```python
from build123d import *

# Parameters (mm, degrees)
SKETCH1_R             = 60.5
BOSS_EXTRUDE1_DEPTH   = 4
SKETCH2_R             = 12
CUT_EXTRUDE1_DEPTH    = 4
F_3_0MM_DOWEL_HOLE1_D = 3
SKETCH6_W             = 4
SKETCH6_H             = 46
CUT_EXTRUDE2_DEPTH    = 4


with BuildPart() as part:
    # Sketch1 → Boss-Extrude1 (new body)
    with BuildSketch(Plane(origin=(0, 0, 0), x_dir=(1, 0, 0), z_dir=(0, 1, 0))):
        with Locations(Location((0, 0, 0), (0, 0, 270))):
            Circle(SKETCH1_R)
    extrude(amount=BOSS_EXTRUDE1_DEPTH)

    # Sketch2 → Cut-Extrude1 (cut)
    with BuildSketch(Plane(origin=(0, 4, 0), x_dir=(1, 0, 0), z_dir=(0, 1, 0))):
        with Locations(Location((0, -20, 0), (0, 0, 270))):
            Circle(SKETCH2_R)
        with Locations(Location((13, 12, 0), (0, 0, 270))):
            Circle(SKETCH2_R)
        with Locations(Location((-13, 12, 0), (0, 0, 270))):
            Circle(SKETCH2_R)
    extrude(amount=-CUT_EXTRUDE1_DEPTH, mode=Mode.SUBTRACT)

    # Ø3.0mm Dowel Hole1 (through all)
    with Locations(Plane(origin=(-22.5, 4, -24), x_dir=(0, 0, 1), z_dir=(0, 1, 0))):
        with Locations((0, 0), (24, 19), (0, 26), (24, 45), (32, 13), (56, 32)):
            Hole(F_3_0MM_DOWEL_HOLE1_D / 2)

    # Sketch6 → Cut-Extrude2 (cut)
    with BuildSketch(Plane(origin=(0, 4, 0), x_dir=(1, 0, 0), z_dir=(0, 1, 0))):
        with Locations((-37, 0)):
            Rectangle(SKETCH6_W, SKETCH6_H)
    cut_extrude2 = extrude(amount=-CUT_EXTRUDE2_DEPTH, mode=Mode.SUBTRACT)

    # Mirror1: Cut-Extrude2 across plane
    add(cut_extrude2.mirror(Plane(origin=(0, 0, 0), x_dir=(0, 0, 1), z_dir=(1, 0, 0))), mode=Mode.SUBTRACT)


solid = part.part
```
For this review, take the finished solid that the model builds, in its own axes (mm). A direction names the side the tool comes from. Coordinates: 2 decimals unless noted, no trailing zeros. Order: outer loops, then holes, each group sorted by start corner. A loop starts at its lowest first (then second) coordinate and runs counter-clockwise, first axis right, second up. Notation, with made-up numbers: (0, 33.25) -> (25, 33.25) arc R25 cw to (25, 61.25) -> close; hole circle Ø9 at (25.5, -20.75). An arc over 180 degrees is marked (long way). Answer as CSV lines item,"result".
Q1. We need section C-C (x = 3.5). State the section outline as (y, z) points, plus the area to 3 significant figures.
Model answer:
outline,"(0, -60.4) -> (4, -60.4) -> (4, -25.5) -> (0, -25.5) -> close; (0, -22.5) -> (4, -22.5) -> (4, -19.33) -> (0, -19.33) -> close; (0, -4.67) -> (4, -4.67) -> (4, 8.52) -> (0, 8.52) -> close; (0, 31.48) -> (4, 31.48) -> (4, 60.4) -> (0, 60.4) -> close"
area,"321 mm2"
Q2. Clearance check with flat-ended pins moving along their axes: pin 1 Ø6 at (x, z) = (18.5, 41) entering from -Y; pin 2 Ø2 at (y, z) = (3.5, -20) entering from +X; pin 3 Ø1.2 at (y, z) = (3, 6) entering from -X; pin 4 Ø1.5 at (x, y) = (2, 3) entering from +Z. State where each tip first meets the part, or that it passes through.
Model answer:
pin 1,"stops at y = 0"
pin 2,"stops at x = 57.44"
pin 3,"stops at x = -60.26"
pin 4,"stops at z = 60.49"
Q3. Wall thickness on line 1 along X through (y, z) = (0.45, -22); line 2 along X through (y, z) = (3.4, 3); line 3 along Z through (x, y) = (7, 3.15): over which ranges is each line inside the solid? List them lowest first. Write a range as [from, to].
Model answer:
line 1,"x = [-56.36, -39], [-35, -19.63], [-6.37, 6.37], [19.63, 35], [39, 56.36]"
line 2,"x = [-60.43, -39], [-35, 35], [39, 60.43]"
line 3,"z = [-60.09, -22.39], [-1.61, 10.25], [29.75, 60.09]"
Q4. We need section D-D (z = 26). State the section outline as (x, y) points.
Model answer:
outline,"(-54.63, 0) -> (-10.39, 0) -> (-10.39, 4) -> (-54.63, 4) -> close; (10.39, 0) -> (54.63, 0) -> (54.63, 4) -> (10.39, 4) -> close"
Q5. We need section A-A (y = 1.8). Count the separate pieces of the cut face and the enclosed holes in it, plus the area to 3 significant figures.
Model answer:
separate pieces,"1"
enclosed holes,"11"
area,"9,730 mm2"
Q6. For faces 1 (the face through (1, 4, -1)), 2 (the face through (39, 2, 0)), list the 3-axis set-ups (+Z, -Z, +X, -X, +Y, -Y) from which the entire face can be reached by the end or side of a thin tool; tool diameter is ignored.
Model answer:
face 1,"+Z, -Z, +X, -X, +Y"
face 2,"+Y, -Y"
Q7. We need section B-B (z = -12). State the section outline as (x, y) points, plus the area to 3 significant figures.
Model answer:
outline,"(-59.3, 0) -> (-39, 0) -> (-39, 4) -> (-59.3, 4) -> close; (-35, 0) -> (-25, 0) -> (-25, 4) -> (-35, 4) -> close; (-1, 0) -> (1, 0) -> (1, 4) -> (-1, 4) -> close; (25, 0) -> (35, 0) -> (35, 4) -> (25, 4) -> close; (39, 0) -> (59.3, 0) -> (59.3, 4) -> (39, 4) -> close"
area,"250 mm2"
Q8. Draft analysis for pull direction Z (two halves, no side actions). For faces 3 (the face through (-59.06, 1.97, -13.12)), 4 (the face through (-2, 2, 0)), 5 (the face through (1, 0, -1)), state which applies: released by +Z, released by -Z, zero draft, split by the parting line, or undercut.
Model answer:
face 3,"split by the parting line"
face 4,"undercut"
face 5,"zero draft"
